Geometry: final body of the model. Coordinates: model frame, mm. Face numbers are marked on the shaded views. A direction names the side the tool comes from. Coordinates: 2 decimals unless noted, no trailing zeros. Order: outer loops, then holes, each group sorted by start corner. A loop starts at its lowest first (then second) coordinate and runs counter-clockwise, first axis right, second up. Notation, with made-up numbers: (32, 88) - (59, 88) arc R8 cw to (59, 95) - close; hole circle Ø2 at (-23, 49.5). An arc over 180 degrees is marked (long way). Use a Markdown table: item, result. Add a question column.
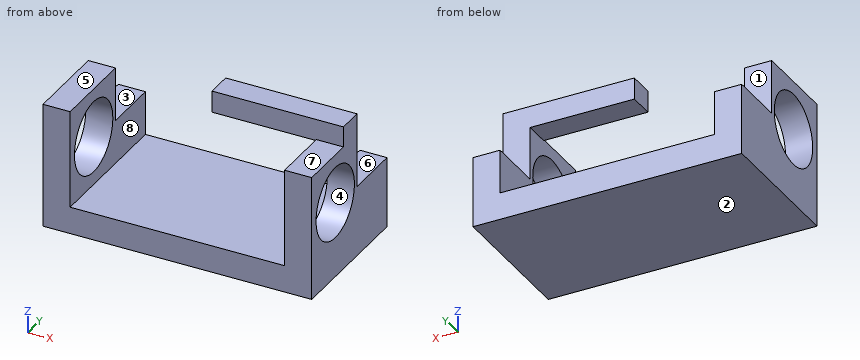
```python
from build123d import *

# Parameters (mm, degrees)
CROQUIS2_W              = 49.5
CROQUIS2_H              = 26.9
SALIENTE_EXTRUIR1_DEPTH = 26.1
CORTAR_EXTRUIR2_DEPTH   = 26.1
CORTAR_EXTRUIR3_REACH   = 64.089
CROQUIS3_W              = 13.8
CROQUIS3_H              = 10.4
CORTAR_EXTRUIR4_REACH   = 60.181
CROQUIS9_R              = 6.65
CORTAR_EXTRUIR5_REACH   = 64.089
CROQUIS8_R              = 6.65
CORTAR_EXTRUIR6_DEPTH   = 10.4
CROQUIS10_W             = 24.2
CROQUIS10_H             = 11
CORTAR_EXTRUIR7_DEPTH   = 3.8
CROQUIS13_W             = 19.2
CROQUIS13_H             = 11
CORTAR_EXTRUIR8_DEPTH   = 0.2
CORTAR_EXTRUIR9_REACH   = 64.089
CROQUIS14_W             = 3.8
CROQUIS14_H             = 15.7
CROQUIS16_W             = 4
CROQUIS16_H             = 4.7
SALIENTE_EXTRUIR2_DEPTH = 19.2
CROQUIS17_W             = 3.8
CROQUIS17_H             = 4.7
SALIENTE_EXTRUIR3_DEPTH = 5
CORTAR_EXTRUIR10_REACH  = 60.326


with BuildPart() as part:
    # Croquis2 → Saliente-Extruir1 (new body)
    with BuildSketch(Plane(origin=(0, 0, 0), x_dir=(1, 0, 0), z_dir=(0, 1, 0))):
        with Locations((-24.75, -13.45)):
            Rectangle(CROQUIS2_W, CROQUIS2_H)
    extrude(amount=SALIENTE_EXTRUIR1_DEPTH)

    # Croquis6 → Cortar-Extruir2 (cut)
    with BuildSketch(Plane(origin=(0, 26.1, 0), x_dir=(1, 0, 0), z_dir=(0, 1, 0))):
        Polygon((-44.5, -21.9), (-44.5, -22.9), (-25.3, -22.9), (-25.3, -26.9), (-5, -26.9), (-5, -21.9), (-5, -5), (-44.5, -5), align=None)
    extrude(amount=-CORTAR_EXTRUIR2_DEPTH, mode=Mode.SUBTRACT)

    # Croquis3 → Cortar-Extruir3 (cut, up to next)
    with BuildSketch(Plane(origin=(0, 0, 0), x_dir=(0, 0, -1), z_dir=(1, 0, 0)), mode=Mode.PRIVATE) as cortar_extruir3_sk1:
        with Locations((-20, 20.9)):
            Rectangle(CROQUIS3_W, CROQUIS3_H)
    cortar_extruir3_tool1 = extrude(cortar_extruir3_sk1.sketch, amount=-CORTAR_EXTRUIR3_REACH, mode=Mode.PRIVATE) & part.part
    add(cortar_extruir3_tool1.solids().sort_by_distance((0, 20.9, 20))[0], mode=Mode.SUBTRACT)

    # Croquis9 → Cortar-Extruir4 (cut, up to next)
    with BuildSketch(Plane(origin=(-44.5, 0, 0), x_dir=(0, 0, -1), z_dir=(1, 0, 0)), mode=Mode.PRIVATE) as cortar_extruir4_sk1:
        with Locations((-14.05, 8.15)):
            Circle(CROQUIS9_R)
    cortar_extruir4_tool1 = extrude(cortar_extruir4_sk1.sketch, amount=-CORTAR_EXTRUIR4_REACH, mode=Mode.PRIVATE) & part.part
    add(cortar_extruir4_tool1.solids().sort_by_distance((-44.5, 8.15, 14.05))[0], mode=Mode.SUBTRACT)

    # Croquis8 → Cortar-Extruir5 (cut, up to next)
    with BuildSketch(Plane(origin=(0, 0, 0), x_dir=(0, 0, -1), z_dir=(1, 0, 0)), mode=Mode.PRIVATE) as cortar_extruir5_sk1:
        with Locations((-14.05, 8.15)):
            Circle(CROQUIS8_R)
    cortar_extruir5_tool1 = extrude(cortar_extruir5_sk1.sketch, amount=-CORTAR_EXTRUIR5_REACH, mode=Mode.PRIVATE) & part.part
    add(cortar_extruir5_tool1.solids().sort_by_distance((0, 8.15, 14.05))[0], mode=Mode.SUBTRACT)

    # Croquis11 → Cortar-Extruir6 (cut)
    with BuildSketch(Plane(origin=(0, 26.1, 0), x_dir=(1, 0, 0), z_dir=(0, 1, 0))):
        Polygon((-44.5, -13.1), (-49.5, -13.1), (-49.5, -26.9), (-25.3, -26.9), (-25.3, -22.9), (-44.5, -22.9), align=None)
    extrude(amount=-CORTAR_EXTRUIR6_DEPTH, mode=Mode.SUBTRACT)

    # Croquis10 → Cortar-Extruir7 (cut)
    with BuildSketch(Plane.XY.offset(26.9)):
        with Locations((-37.4, 5.5)):
            Rectangle(CROQUIS10_W, CROQUIS10_H)
    extrude(amount=-CORTAR_EXTRUIR7_DEPTH, mode=Mode.SUBTRACT)

    # Croquis13 → Cortar-Extruir8 (cut)
    with BuildSketch(Plane(origin=(0, 0, 22.9), x_dir=(-1, 0, 0), z_dir=(0, 0, -1))):
        with Locations((34.9, 5.5)):
            Rectangle(CROQUIS13_W, CROQUIS13_H)
    extrude(amount=-CORTAR_EXTRUIR8_DEPTH, mode=Mode.SUBTRACT)

    # Croquis14 → Cortar-Extruir9 (cut, up to next)
    with BuildSketch(Plane(origin=(0, 0, 0), x_dir=(0, 0, -1), z_dir=(1, 0, 0)), mode=Mode.PRIVATE) as cortar_extruir9_sk1:
        with Locations((-25, 7.85)):
            Rectangle(CROQUIS14_W, CROQUIS14_H)
    cortar_extruir9_tool1 = extrude(cortar_extruir9_sk1.sketch, amount=-CORTAR_EXTRUIR9_REACH, mode=Mode.PRIVATE) & part.part
    add(cortar_extruir9_tool1.solids().sort_by_distance((0, 7.85, 25))[0], mode=Mode.SUBTRACT)

    # Croquis16 → Saliente-Extruir2 (add)
    with BuildSketch(Plane.ZY.offset(5)):
        with Locations((24.9, 13.35)):
            Rectangle(CROQUIS16_W, CROQUIS16_H)
    extrude(amount=SALIENTE_EXTRUIR2_DEPTH)

    # Croquis17 → Saliente-Extruir3 (add)
    with BuildSketch(Plane(origin=(-5, 0, 0), x_dir=(0, 0, -1), z_dir=(1, 0, 0))):
        with Locations((-25, 13.35)):
            Rectangle(CROQUIS17_W, CROQUIS17_H)
    extrude(amount=SALIENTE_EXTRUIR3_DEPTH)

    # Croquis18 → Cortar-Extruir10 (cut, up to next)
    with BuildSketch(Plane.XZ.offset(-11), mode=Mode.PRIVATE) as cortar_extruir10_sk1:
        Polygon((-25.3, 26.9), (-49.5, 26.9), (-49.5, 23.1), (-44.5, 23.1), (-44.5, 22.9), (-25.3, 22.9), align=None)
    cortar_extruir10_tool1 = extrude(cortar_extruir10_sk1.sketch, amount=-CORTAR_EXTRUIR10_REACH, mode=Mode.PRIVATE) & part.part
    add(cortar_extruir10_tool1.solids().sort_by_distance((-37.299791, 11, 24.919833))[0], mode=Mode.SUBTRACT)


solid = part.part
```
1) Draft query along Z for the marked faces 1, 2, 3 and 4. Return one class per face: released by +Z, released by -Z, zero draft, split by the parting line, or undercut.
2) Section query D-D (y = 16.5). Return the cut outline in (x, z).
3) Line query: line 1 (Y direction, x = -47.25, z = 14.05); line 2 (X direction, y = 16.75, z = 9.25); line 3 (Z direction, x = -36, y = 16.5). Output: solid intervals per line, ascending. Write a range as from..to.
4) Access query for the marked faces 5, 6, 7 and 8. Directions: +Z, -Z, +X, -X, +Y, -Y. A direction counts if a zero-diameter tool reaches every point of the face in a straight line with its end or side. Return the directions, or none.
5) First-contact query: pin 1 (11 mm diameter, centred on x = -9.5, z = 17, fed in from +Y); pin 2 (2.5 mm diameter, centred on x = -48, y = 21, fed in from +Z); pin 3 (5.5 mm diameter, centred on x = -46, y = 11.5, fed in from +Z). Flat tips, straight axial feed; report the tip coordinate or a pass-through.
6) Section query A-A (y = 8.15). Return the cut outline in (x, z).
7) Section query B-B (z = 14.05). Return the cut outline in (x, y).
8) Section query C-C (x = -20.5). Return the cut outline in (y, z), and give its area (3 significant figures).
From the geometry:
| question | item | result |
|---|---|---|
| 1 | face 1 | zero draft |
| 1 | face 2 | released by -Z |
| 1 | face 3 | released by +Z |
| 1 | face 4 | undercut |
| 2 | outline | (-49.5, 0) - (0, 0) - (0, 13.1) - (-5, 13.1) - (-5, 5) - (-44.5, 5) - (-44.5, 13.1) - (-49.5, 13.1) - close |
| 3 | line 1 | y = 0..1.5, 14.8..15.7 |
| 3 | line 2 | x = -49.5..-44.5, -5..0 |
| 3 | line 3 | z = 0..5 |
| 4 | face 5 | +Z, -X, +Y, -Y |
| 4 | face 6 | +Z, +X, -X, +Y |
| 4 | face 7 | +Z, +X, -X, -Y |
| 4 | face 8 | +Z, +Y, -Y |
| 5 | pin 1 | stops at y = 15.7 |
| 5 | pin 2 | stops at z = 13.1 |
| 5 | pin 3 | stops at z = 23.1 |
| 6 | outline | (-49.5, 0) - (0, 0) - (0, 7.4) - (-5, 7.4) - (-5, 5) - (-44.5, 5) - (-44.5, 7.4) - (-49.5, 7.4) - close; (-49.5, 20.7) - (-44.5, 20.7) - (-44.5, 23.1) - (-49.5, 23.1) - close; (-5, 20.7) - (0, 20.7) - (0, 23.1) - (-5, 23.1) - close |
| 7 | outline | (-49.5, 0) - (-44.5, 0) - (-44.5, 1.5) - (-49.5, 1.5) - close; (-49.5, 14.8) - (-44.5, 14.8) - (-44.5, 15.7) - (-49.5, 15.7) - close; (-5, 0) - (0, 0) - (0, 1.5) - (-5, 1.5) - close; (-5, 14.8) - (0, 14.8) - (0, 15.7) - (-5, 15.7) - close |
| 8 | outline | (0, 0) - (26.1, 0) - (26.1, 5) - (0, 5) - close; (11, 22.9) - (15.7, 22.9) - (15.7, 26.9) - (11, 26.9) - close |
| 8 | area | 149 mm^2 |
